```python
from build123d import *

# Parameters (mm, degrees)
BOSS_EXTRUDE1_DEPTH        = 5
F_3_3_3_3_DIAMETER_HOLE1_D = 3.3


with BuildPart() as part:
    # Sketch1 → Boss-Extrude1 (new body)
    with BuildSketch(Plane(origin=(0, 0, 0), x_dir=(1, 0, 0), z_dir=(0, 1, 0))):
        Polygon((-43, 60), (-43, 35), (30, 35), (30, 60), (60, 60), (60, 36), (35, 36), (35, -36), (60, -36), (60, -60), (30, -60), (30, -35), (-43, -35), (-43, -60), (-60, -60), (-60, 60), align=None)
    extrude(amount=BOSS_EXTRUDE1_DEPTH)

    # Ø3.3 (3.3) Diameter Hole1 (through all)
    with Locations(Plane(origin=(0, 5, 0), x_dir=(1, 0, 0), z_dir=(0, 1, 0))):
        with Locations((-45, 45), (45, 45), (45, -45), (-45, -45)):
            Hole(F_3_3_3_3_DIAMETER_HOLE1_D / 2)


solid = part.part
```
Source: CAD feature listing. Evaluate the final solid. Frame: model axes, mm. A direction names the side the tool comes from. Coordinates: 2 decimals unless noted, no trailing zeros. Write each loop counter-clockwise with the first axis right and the second up, starting at its lowest first coordinate (ties: lowest second). Pieces come first, ordered by that corner, then holes. Notation, with made-up numbers: (68, 79.5) -> (103, 79.5) arc R23 cw to (103, 96.5) -> close; hole circle Ø3 at (32, 89.25). An arc over 180 degrees is marked (long way). Return JSON: item names as keys, results as strings. Group by question number.
1) Set-up query: faces 1 (the face through (35, 2, -1)), 2 (the face through (30, 2, -47)), 3 (the face through (-43.784, 2.465, -46.115)), 4 (the face through (-60, 2, 1)), 5 (the face through (-43, 2, 47)). Return all of +Z, -Z, +X, -X, +Y, -Y with unobstructed straight access to the full face (end or side cutting, diameter ignored); none if empty.
2) Contact query for flat-ended pins moving along their axis: P1, Ø1.5, axis at y = 3.5, z = 5.5, coming from the +X side; P2, Ø2.5, axis at x = -4, y = 2.5, coming from the +Z side. Output: stop coordinate, or through.
3) Section query D-D, the plane z = 45. Return loops of the section in (x, y), plus the area to 3 significant figures.
4) Section query A-A, the plane x = -45. Return loops of the section in (y, z), plus the area to 3 significant figures.
5) Section query B-B, the plane x = 45. Return loops of the section in (y, z), plus the area to 3 significant figures.
6) Ray query, line 1 along X through (y, z) = (1.7, -45); line 2 along Z through (x, y) = (-45, 1.25); line 3 along X through (y, z) = (1.95, 48). Return the intervals inside material, ascending.
7) Section query C-C, the plane y = 1.85. Return loops of the section in (x, z), plus the area to 3 significant figures.
8) Mould query, pull axis Z, two halves, no side actions, for faces 6 (the face through (30, 2, 48)), 7 (the face through (45, 2, -60)), 8 (the face through (47, 2, 36)), 9 (the face through (48, 2, -36)). Classes: +Z half, -Z half, draft (parallel to the pull), parting line (faces both ways), or undercut.
From the geometry:
{
 "1": {"face 1": "+X, +Y, -Y", "face 2": "-Z, +Y, -Y", "face 3": "+Y, -Y", "face 4": "+Z, -Z, -X, +Y, -Y", "face 5": "+Z, +Y, -Y"},
 "2": {"P1": "x = 35", "P2": "z = 35"},
 "3": {"outline": "(-60, 0) -> (-46.65, 0) -> (-46.65, 5) -> (-60, 5) -> close; (-43.35, 0) -> (-43, 0) -> (-43, 5) -> (-43.35, 5) -> close; (30, 0) -> (43.35, 0) -> (43.35, 5) -> (30, 5) -> close; (46.65, 0) -> (60, 0) -> (60, 5) -> (46.65, 5) -> close", "area": "202 mm²"},
 "4": {"outline": "(0, -60) -> (5, -60) -> (5, -46.65) -> (0, -46.65) -> close; (0, -43.35) -> (5, -43.35) -> (5, 43.35) -> (0, 43.35) -> close; (0, 46.65) -> (5, 46.65) -> (5, 60) -> (0, 60) -> close", "area": "567 mm²"},
 "5": {"outline": "(0, -60) -> (5, -60) -> (5, -46.65) -> (0, -46.65) -> close; (0, -43.35) -> (5, -43.35) -> (5, -36) -> (0, -36) -> close; (0, 36) -> (5, 36) -> (5, 43.35) -> (0, 43.35) -> close; (0, 46.65) -> (5, 46.65) -> (5, 60) -> (0, 60) -> close", "area": "207 mm²"},
 "6": {"line 1": "-60 to -46.65, -43.35 to -43, 30 to 43.35, 46.65 to 60", "line 2": "-60 to -46.65, -43.35 to 43.35, 46.65 to 60", "line 3": "-60 to -43, 30 to 60"},
 "7": {"outline": "(-60, -60) -> (-43, -60) -> (-43, -35) -> (30, -35) -> (30, -60) -> (60, -60) -> (60, -36) -> (35, -36) -> (35, 36) -> (60, 36) -> (60, 60) -> (30, 60) -> (30, 35) -> (-43, 35) -> (-43, 60) -> (-60, 60) -> close; hole circle Ø3.3 at (-45, -45); hole circle Ø3.3 at (-45, 45); hole circle Ø3.3 at (45, -45); hole circle Ø3.3 at (45, 45)", "area": "8,920 mm²"},
 "8": {"face 6": "draft", "face 7": "-Z half", "face 8": "undercut", "face 9": "undercut"}
}
